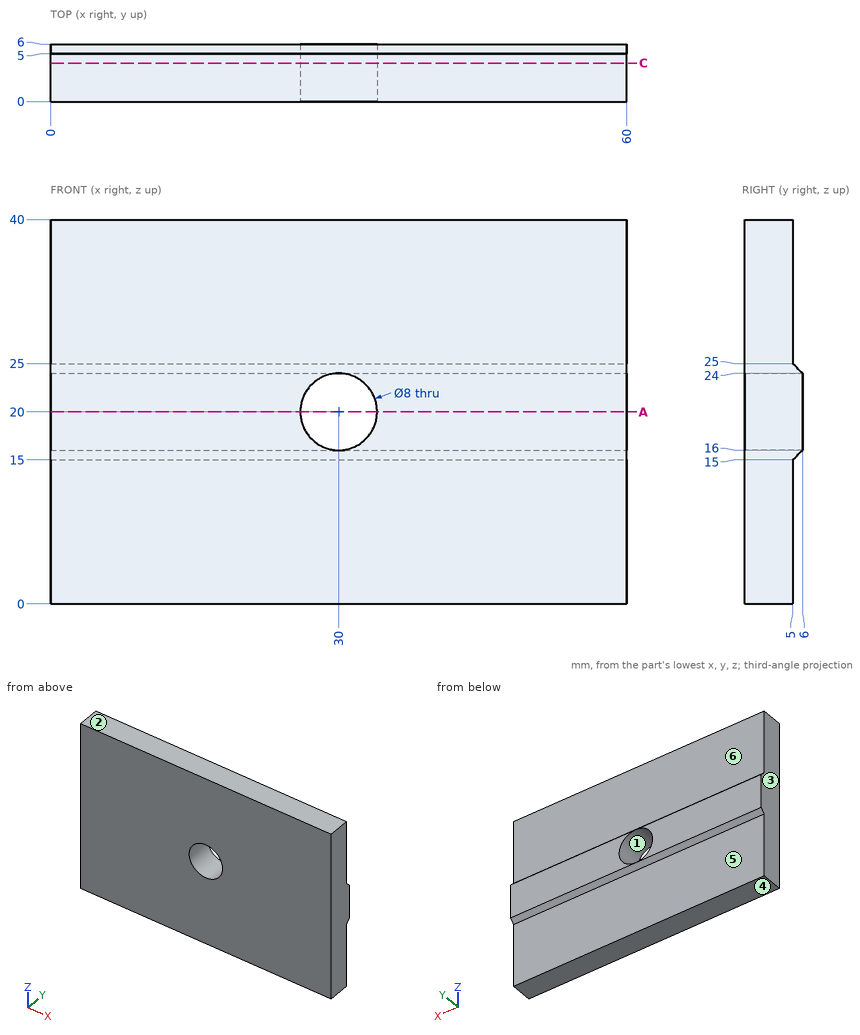
Can you work these out from the drawing? Everything is in mm from the part's minimum corner. A direction names the side the tool comes from. Round coordinates to 2 decimals unless told otherwise and drop trailing zeros. Loops run counter-clockwise (first coordinate to the right, second up) from the corner with the lowest first, then second, coordinate; pieces in that order, holes last. Notation, with made-up numbers: (-29.5, -39) -> (-19.5, -39) arc R15 cw to (-19.5, -35) -> close; hole circle Ø2 at (57, 4.25). An arc over 180 degrees is marked (long way). One line per question, with ' | ' between items.
(1) If we section it at C-C on y = 4: List the corners of the cut face in (x, z) for me, and give its area (3 significant figures).
Model answer:
outline: (0, 0) -> (60, 0) -> (60, 40) -> (0, 40) -> close; hole circle Ø8 at (30, 20) | area: 2,350 mm^2
(2) Thinking about a two-plate mould opening in X: for the marked faces 1, 2 and 3, which applies, released by +X, released by -X, zero draft, split by the parting line, or undercut?
Model answer:
face 1: undercut | face 2: zero draft | face 3: released by -X
(3) If we section it at A-A on z = 20: List the corners of the cut face in (x, y) for me, and give its area (3 significant figures).
Model answer:
outline: (0, 0) -> (26, 0) -> (26, 6) -> (0, 6) -> close; (34, 0) -> (60, 0) -> (60, 6) -> (34, 6) -> close | area: 312 mm^2
(4) For pin 1 Ø12 at (x, z) = (20, 35) entering from +Y, with a flat end and sliding along its axis, tell me the tip position at first contact or that it passes through.
Model answer:
pin 1: stops at y = 5
(5) If I drill on probe 1 along X at (y, z) = (2.05, 20); probe 2 along Z at (x, y) = (30, 4.7); probe 3 along Y at (x, z) = (34, 28.5), over which ranges is the centre line in solid material (lowest first)?
Model answer:
probe 1: x = 0 to 26, 34 to 60 | probe 2: z = 0 to 16, 24 to 40 | probe 3: y = 0 to 5
(6) For the marked faces 4, 5 and 6, which set-ups out of +Z, -Z, +X, -X, +Y, -Y let a thin tool reach every point of the face, with its end or its side?
Model answer:
face 4: -Z, +X, -X, +Y, -Y | face 5: -Z, +X, -X, +Y | face 6: +Z, +X, -X, +Y
